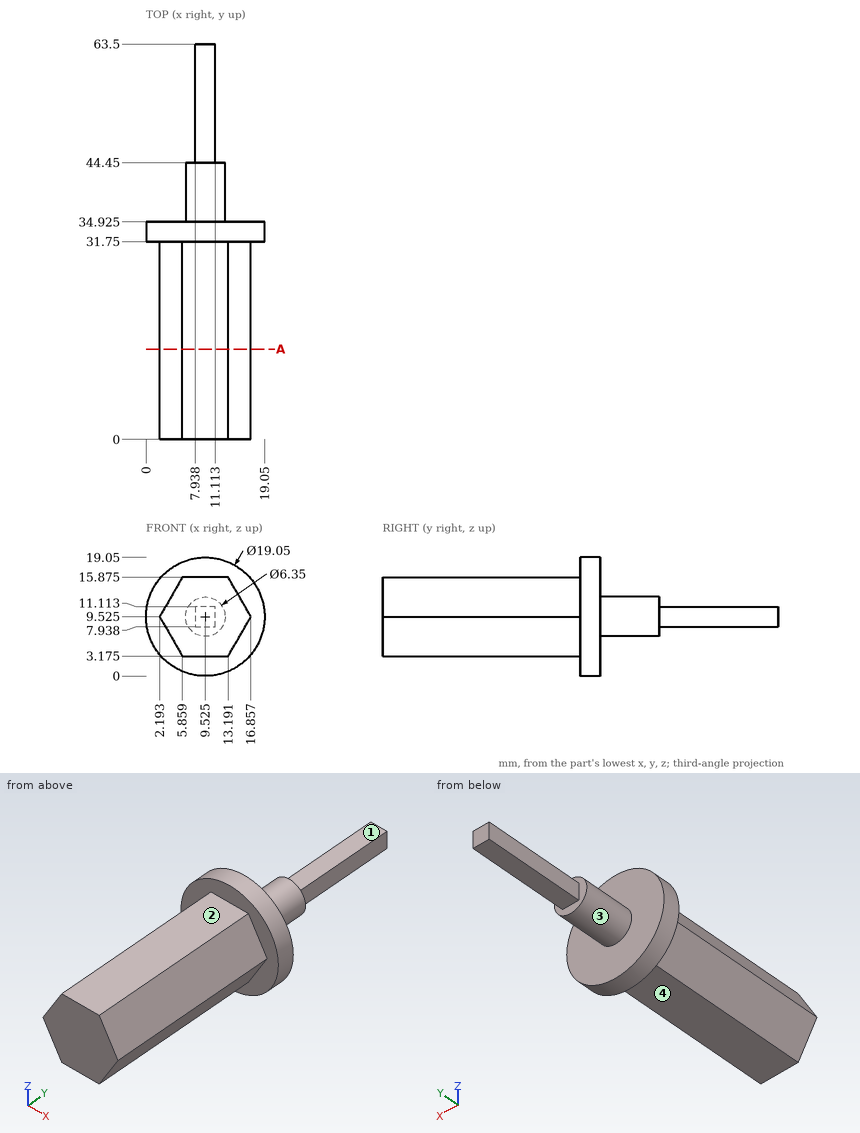
Input: dimensioned drawing with shaded views. Units: mm. Origin: part minimum x, y, z. A direction names the side the tool comes from. Coordinates: 2 decimals unless noted, no trailing zeros. Loops run counter-clockwise (first coordinate to the right, second up) from the corner with the lowest first, then second, coordinate; pieces in that order, holes last. Notation, with made-up numbers: M 52.25,20 L 111.25,20 A37 cw 111.25,59 Z; hole C 81.5,79 d1. An arc over 180 degrees is marked long. One line per item, written item: value. Start each with the question number.
1) Material intervals for L1, parallel to Z at x = 6.5, y = 14.5 (1 decimal); L2, parallel to Z at x = 10.75, y = 48.5; L3, parallel to Y at x = 8.25, z = 4.25 (1 decimal), sorted ascending. Write a range as from..to.
2) Cut plane A-A (y = 14.5). Return loops of the section in (x, z) (1 decimal), then the cut area to 3 significant figures.
3) Reachability of the marked faces 1, 2, 3 and 4 from +Z, -Z, +X, -X, +Y, -Y: full face, straight path, thin tool, end or side. Return the list, or none.
4) Pin query (flat end, axial travel): P1, Ø6, axis at x = 9, y = 8.5, coming from the -Z side (1 decimal); P2, Ø3, axis at y = 25.5, z = 3, coming from the +X side (1 decimal); P3, Ø1.6, axis at x = 10, y = 58, coming from the -Z side. Return the tip coordinate at first contact, or that it passes through.
Evaluation:
1. L1: 3.2..15.9
1. L2: 7.94..11.11
1. L3: 0..34.9
2. outline: M 2.2,9.5 L 5.9,3.2 L 13.2,3.2 L 16.9,9.5 L 13.2,15.9 L 5.9,15.9 Z
2. area: 140 mm^2
3. face 1: +Z, +X, -X, +Y
3. face 2: +Z, +X, -X, -Y
3. face 3: +Y
3. face 4: -Z, +X, -X, -Y
4. P1: z = 3.2
4. P2: x = 14
4. P3: z = 7.94
